Autodesk Inventor part; units mm, degrees
ref_plane "Plano de trabajo1" through (0, 3.925, -4) normal (0, 1, 0) x (-1, 0, 0)
ref_plane "YZ Plane" through (0, 0, 0) normal (1, 0, 0) x (0, 1, 0)
ref_plane "XY Plane" through (0, 0, 0) normal (0, 0, 1) x (1, 0, 0)
sketch "Boceto1" plane through (0, 0, 0) normal (0, 0, 1) x (1, 0, 0)
  circle A0 centre (0, 0) radius 13.5
  dimension "d0" = 27
extrude "Extrusión1" add sketch "Boceto1" along normal blind 2
sketch "Boceto2" plane through (0, 0, 0) normal (0, 0, -1) x (-1, 0, 0)
  circle A0 centre (0, 0) radius 13.5
  circle A1 centre (0, 0) radius 11.23
  dimension "d3" = 22.46
extrude "Extrusión2" add sketch "Boceto2" along normal blind 2 contours A1
sketch "Boceto3" plane through (0, 0, -2) normal (0, 0, -1) x (-1, 0, 0)
  circle A0 centre (0, 0) radius 11.23
  circle A1 centre (0, 0) radius 5.92
  dimension "d6" = 11.84
extrude "Extrusión3" add sketch "Boceto3" along normal blind 2 contours A1
sketch "Boceto4" plane through (0, 0, -4) normal (0, 0, -1) x (-1, 0, 0)
  circle A0 centre (0, 0) radius 5.92
  circle A1 centre (0, 0) radius 3.925
  dimension "d9" = 7.85
extrude "Extrusión4" add sketch "Boceto4" along normal blind 2.5 contours A1
hole "Hole1" at (0, 0, 2) direction (0, 0, -1) diameter 2.02 end through all
hole "Hole2" at (0, 0, -6.5) direction (0, 0, 1) diameter 5.2 depth 2.5
ref_plane "Plano de trabajo1" through (0, 3.925, -4) normal (0, 1, 0) x (-1, 0, 0)
sketch "Boceto11" plane through (0, 3.925, -4) normal (0, 1, 0) x (-1, 0, 0)
  line L0 (0, 9) -> (0, -15.4341)
  line L1 (1.14, 0) -> (-1.14, 0)
  line L2 (-1.14, 0) -> (-1.14, -2.5)
  line L3 (-1.14, -2.5) -> (1.14, -2.5)
  line L4 (1.14, -2.5) -> (1.14, 0)
  dimension "d44" = 2.28
  dimension "d45" = 2.5
  dimension "d46" = 1.14
extrude "Extrusión6" add sketch "Boceto11" along normal blind 1.5 and the other way blind 1
sketch "Boceto13" plane through (0, 0, -2) normal (0, 0, -1) x (-1, 0, 0)
  circle A0 centre (0, 7.4449) radius 1
extrude "Extrusión7" cut sketch "Boceto13" against normal blind 6.5
pattern_circular "Patrón circular2" count 4 over 360 about axis through (0, 0, -10) along (0, 0, 1) of "Extrusión7"
hole "Hole6" at (-7.4449, 0, -4) direction (0, 0, 1) diameter 5.43 depth 2
mirror "Simetría2" about plane through (0, 0, 0) normal (1, 0, 0) of "Hole6"
properties part number "TapaPosterior"
The listing builds one solid part. Answer for the finished solid, in the listing's coordinates (mm). A direction names the side the tool comes from. Coordinates: 2 decimals unless noted, no trailing zeros. Loops run counter-clockwise (first coordinate to the right, second up) from the corner with the lowest first, then second, coordinate; pieces in that order, holes last. Notation, with made-up numbers: (-11.5, -31.5) -> (27.5, -31.5) arc R15 ccw to (27.5, -23.5) -> close; hole circle Ø2 at (-20.75, -39). An arc over 180 degrees is marked (long way). Use one line per item in the form item = value. Start each with the question number.
Item 1: The part is cut by section A-A on x = 0. Count the separate pieces of the cut face and the enclosed holes in it, then the cut area to 3 significant figures.
Item 2: The mould has two halves that part along Y. Classify faces 1 (the face through (-0.16, -3.92, -5.23)), 2 (the face through (0, 3, -6.5)), 3 (the face through (-0.1, -5.92, -2.99)), 4 (the face through (-2.578, -0.338, -5.232)): released by +Y, released by -Y, zero draft, split by the parting line, or undercut.
Item 3: The part is cut by section D-D on y = 9.5. Determine the outline of the cut face in (x, z).
Item 4: A tool of negligible diameter and unlimited length cuts with its end or side. For faces 5 (the face through (-1.14, 5, -5)), 6 (the face through (4.73, 0.03, -2.99)), 7 (the face through (0, 5.425, -5)), 8 (the face through (1, 1, -4)), 9 (the face through (-4.73, -0.03, -2.99)), from which of +Z, -Z, +X, -X, +Y, -Y can it reach the whole face along a straight path? Write none if from no direction.
Item 5: The part is cut by section C-C on x = -3.5. Determine the outline of the cut face in (y, z).
Item 6: Consider L1, parallel to Y at x = 0, z = -0.95; L2, parallel to X at y = 0, z = -5.65 (3 decimals); L3, parallel to X at y = -0.5, z = -1.75. Determine where each line is inside the solid, lowest interval first. Write a range as [from, to].
Item 7: The part is cut by section B-B on z = -0.5. Determine the outline of the cut face in (x, y).
Item 8: Flat-ended cylindrical pins translate along their axes: pin 1 Ø1 at (x, y) = (-3.5, -3.5) entering from -Z; pin 2 Ø4 at (y, z) = (1.5, -5) entering from -X; pin 3 Ø1.8 at (x, y) = (0, -7.44) entering from -Z; pin 4 Ø4 at (x, y) = (10, -2.5) entering from -Z. Find the tip coordinate at first contact, or state that the pin passes through.
Answer key:
q1.separate_pieces = 4
q1.enclosed_holes = 0
q1.area = 105 mm2
q2.face_1 = split by the parting line
q2.face_2 = zero draft
q2.face_3 = released by -Y
q2.face_4 = undercut
q3.outline = (-9.59, 0) -> (-5.99, 0) -> (-5.99, -2) -> (5.99, -2) -> (5.99, 0) -> (9.59, 0) -> (9.59, 2) -> (-9.59, 2) -> close
q4.face_5 = -Z, -X, +Y
q4.face_6 = -Z, +X
q4.face_7 = -Z, +X, -X, +Y
q4.face_8 = -Z
q4.face_9 = -Z, -X
q5.outline = (-13.04, 0) -> (-10.67, 0) -> (-10.67, -2) -> (-4.77, -2) -> (-4.77, -4) -> (-1.78, -4) -> (-1.78, -6.5) -> (1.78, -6.5) -> (1.78, -4) -> (4.77, -4) -> (4.77, -2) -> (10.67, -2) -> (10.67, 0) -> (13.04, 0) -> (13.04, 2) -> (-13.04, 2) -> close
q6.L1 = [-11.23, -8.44], [-6.44, -1.01], [1.01, 6.44], [8.44, 11.23]
q6.L2 = [-3.925, -2.6], [2.6, 3.925]
q6.L3 = [-11.22, -8.31], [-6.58, -0.88], [0.88, 6.58], [8.31, 11.22]
q7.outline = circle Ø22.46 at (0, 0); hole circle Ø2 at (-7.44, 0); hole circle Ø2.02 at (0, 0); hole circle Ø2 at (0, -7.44); hole circle Ø2 at (0, 7.44); hole circle Ø2 at (7.44, 0)
q8.pin_1 = -4
q8.pin_2 = -5.58
q8.pin_3 = through
q8.pin_4 = -2
